from build123d import *

# Parameters (mm, degrees)
F2_R            = 19.0246
F3_DEPTH        = 53.849
F4_R            = 6.35
F5_DEPTH        = 53.849
F5_COPIES_COUNT = 4
F6_R            = 3.048


# Not quite as in the source:
# - a pattern or mirror of a feature is missing from the dataset's text; its kind, count and spacing are read off the source's solid


with BuildPart() as f1:
    # F0 (on Right) → F1 (revolve)
    with BuildSketch(Plane.YZ):
        Polygon((34.798, 34.4624179433), (0, 34.925), (0, 0), (53.848, 0), (53.848, 69.85), (34.798, 69.85), align=None)
    revolve(axis=Axis((0, 26.924, 0), (0, 1, 0)))

    # F2 (on Front) → F3 (cut, through all)
    with BuildSketch(Plane.XZ):
        Circle(F2_R)
    extrude(amount=-F3_DEPTH, mode=Mode.SUBTRACT)

    # F4 (on Front) → F5 (cut, through all)
    with BuildSketch(Plane.XZ):
        with Locations((0, 53.848)):
            Circle(F4_R)
    f5 = extrude(amount=-F5_DEPTH, mode=Mode.SUBTRACT)

    # F5_copies: F5 ×4 about axis
    f5_copies_axis = Axis((0, 0, 0), (0, 1, 0))
    for i in range(1, F5_COPIES_COUNT):
        add(f5.rotate(f5_copies_axis, i * 360 / F5_COPIES_COUNT), mode=Mode.SUBTRACT)

    # F6
    f6_edges = [f1.edges().sort_by_distance(p)[0] for p in [
        (0, 0, -34.925),
        (-19.0246, 0, 0),
        (0, 34.798, -69.85),
        (0, 34.798, -34.462418),
    ]]
    fillet(f6_edges, radius=F6_R)


solid = f1.part
Can you work these out from the model? Positions are in its coordinate system, mm. Give positions to 0.01 mm unless a question says otherwise; leave off trailing zeros. Order: outer loops, then holes, each group sorted by start corner. A loop starts at its lowest first (then second) coordinate and runs counter-clockwise, first axis right, second up. Notation, with made-up numbers: M 27,59 L 71,59 A27 cw 71,86 Z; hole C -9.75,77 d1. An arc over 180 degrees is marked long. Use a Markdown table: item, result. Add a question column.
Item 1: Suppose I cut it at A-A (y = 44.5). List the corners of the cut face in (x, z) for me.
Item 2: Suppose I cut it at C-C (y = 30). List the corners of the cut face in (x, z) for me, then the cut area to 3 significant figures.
Item 3: We'd pull the mould along X, two halves only. Please class faces 1 (the conical face through (-21.112, 17.199, -27.534)), 2 (the cylindrical face through (60.144, 44.19, 0.827)), 3 (the flat face through (-29, 34.798, 29)): +X half, -X half, draft (parallel to the pull), parting line (faces both ways), or undercut.
Item 4: Will these pins go through, and if not, where does the flat tip stop? pin 1 (11.5 mm diameter, centred on x = -53.848, z = 0, fed in from -Y); pin 2 (2 mm diameter, centred on y = 31.5, z = 18.5, fed in from -X); pin 3 (3 mm diameter, centred on y = 47.5, z = -33.5, fed in from -X); pin 4 (4 mm diameter, centred on x = 3.5, y = 30, fed in from -Z).
Item 5: If I drill on L1, parallel to X at y = 36.5, z = 1; L2, parallel to X at y = 3, z = 0.5; L3, parallel to Y at x = -44, z = -13, over which ranges is the centre line in solid material (lowest first)? Write a range as [from, to].
Item 6: Suppose I cut it at B-B (y = 12). List the corners of the cut face in (x, z) for me, then the cut area to 3 significant figures.
Answer sheet:
| question | item | result |
|---|---|---|
| 1 | outline | C 0,0 d139.7; hole C -53.85,0 d12.7; hole C 0,0 d38.05; hole C 0,-53.85 d12.7; hole C 0,53.85 d12.7; hole C 53.85,0 d12.7 |
| 2 | outline | C 0,0 d69.05; hole C 0,0 d38.05 |
| 2 | area | 2,610 mm² |
| 3 | face 1 | parting line |
| 3 | face 2 | undercut |
| 3 | face 3 | draft |
| 4 | pin 1 | passes through |
| 4 | pin 2 | stops at x = -29.74 |
| 4 | pin 3 | stops at x = -62.09 |
| 4 | pin 4 | stops at z = -34.5 |
| 5 | L1 | x = [-69.53, -60.12], [-47.58, -19], [19, 47.58], [60.12, 69.53] |
| 5 | L2 | x = [-34.88, -19.02], [19.02, 34.88] |
| 5 | L3 | y = [34.8, 53.85] |
| 6 | outline | C 0,0 d69.53; hole C 0,0 d38.05 |
| 6 | area | 2,660 mm² |
